The listing builds one solid part. Answer for the finished solid, in the listing's coordinates (mm). Face numbers are marked on the shaded views. Coordinates: 2 decimals unless noted, no trailing zeros. Order: outer loops, then holes, each group sorted by start corner. A loop starts at its lowest first (then second) coordinate and runs counter-clockwise, first axis right, second up. Notation, with made-up numbers: (30, 57.25) - (82, 57.25) arc R35 ccw to (82, 95.25) - close; hole circle Ø11 at (-10.5, -8.75). An arc over 180 degrees is marked (long way). Use a Markdown table: item, result. Add a question column.
Item 1: The part is cut by section C-C, the plane y = 7. Give the vertices of the cut face in (x, z), then the cut area to 3 significant figures.
Item 2: Find the intervals of material crossed by line 1 along X through (y, z) = (7.6, 32.7); line 2 along Z through (x, y) = (1.25, 9.75); line 3 along Y through (x, z) = (-4.75, 16), in increasing order.
Item 3: The part is cut by section B-B, the plane z = 28. Give the vertices of the cut face in (x, y), then the cut area to 3 significant figures.
Item 4: The mould has two halves that part along X. Classify the marked faces 1, 2, 3 and 4: released by +X, released by -X, zero draft, split by the parting line, or undercut.
Item 5: The part is cut by section A-A, the plane x = -14.5. Give the vertices of the cut face in (y, z), then the cut area to 3 significant figures.
Item 6: Flat-ended cylindrical pins translate along their axes: P1, Ø4, axis at x = -17.5, z = 34, coming from the -Y side; P2, Ø1, axis at x = -4, z = 20.5, coming from the -Y side; P3, Ø1.5, axis at x = -9.5, z = 22, coming from the -Y side. Find the tip coordinate at first contact, or state that the pin passes through.
Item 7: The part is cut by section D-D, the plane z = 12.7. Give the vertices of the cut face in (x, y), then the cut area to 3 significant figures.
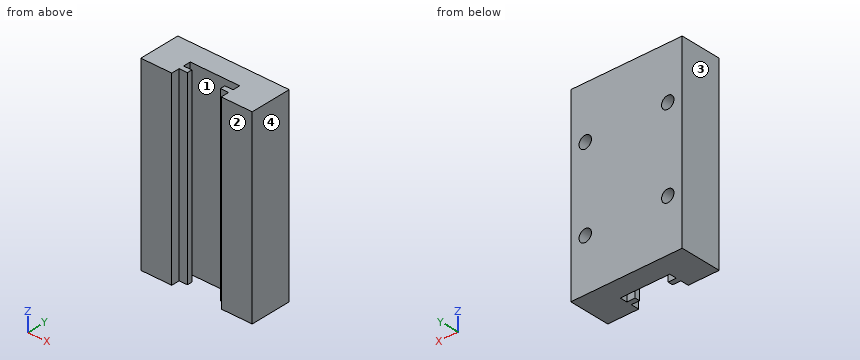
from build123d import *

# Parameters (mm, degrees)
BOSS_EXTRU_1_DEPTH      = 45.4
ESQUISSE2_R             = 1.5
ENL_V_MAT_EXTRU_1_DEPTH = 3.5


with BuildPart() as part:
    # Esquisse1 → Boss.-Extru.1 (new body)
    with BuildSketch(Plane.XY):
        Polygon((-22.795509579, 10), (4.204490421, 10), (4.204490421, 0), (-3.295509579, 0), (-3.295509579, 2), (-5.295509579, 2), (-5.295509579, 3.2), (-3.295509579, 3.2), (-3.295509579, 5), (-15.295509579, 5), (-15.295509579, 3.2), (-13.295509579, 3.2), (-13.295509579, 2), (-15.295509579, 2), (-15.295509579, 0), (-22.795509579, 0), align=None)
    extrude(amount=BOSS_EXTRU_1_DEPTH)

    # Esquisse2 → Enlèv. mat.-Extru.1 (cut)
    with BuildSketch(Plane(origin=(0, 10, 0), x_dir=(1, 0, 0), z_dir=(0, 1, 0))):
        with Locations(Location((-19.295509579, -32.7, 0), (0, 0, 270))):
            Circle(ESQUISSE2_R)
        with Locations(Location((-19.295509579, -12.7, 0), (0, 0, 270))):
            Circle(ESQUISSE2_R)
        with Locations(Location((0.704490421, -12.7, 0), (0, 0, 270))):
            Circle(ESQUISSE2_R)
        with Locations(Location((0.704490421, -32.7, 0), (0, 0, 270))):
            Circle(ESQUISSE2_R)
    extrude(amount=-ENL_V_MAT_EXTRU_1_DEPTH, mode=Mode.SUBTRACT)


solid = part.part
Solution:
| question | item | result |
|---|---|---|
| 1 | outline | (-22.8, 0) - (4.2, 0) - (4.2, 45.4) - (-22.8, 45.4) - close; hole circle Ø3 at (-19.3, 12.7); hole circle Ø3 at (-19.3, 32.7); hole circle Ø3 at (0.7, 12.7); hole circle Ø3 at (0.7, 32.7) |
| 1 | area | 1,200 mm2 |
| 2 | line 1 | x = -22.8 to -20.8, -17.8 to -0.8, 2.2 to 4.2 |
| 2 | line 2 | z = 0 to 11.3, 14.1 to 31.3, 34.1 to 45.4 |
| 2 | line 3 | y = 2 to 3.2, 5 to 10 |
| 3 | outline | (-22.8, 0) - (-15.3, 0) - (-15.3, 2) - (-13.3, 2) - (-13.3, 3.2) - (-15.3, 3.2) - (-15.3, 5) - (-3.3, 5) - (-3.3, 3.2) - (-5.3, 3.2) - (-5.3, 2) - (-3.3, 2) - (-3.3, 0) - (4.2, 0) - (4.2, 10) - (-22.8, 10) - close |
| 3 | area | 215 mm2 |
| 4 | face 1 | undercut |
| 4 | face 2 | zero draft |
| 4 | face 3 | released by -X |
| 4 | face 4 | released by +X |
| 5 | outline | (2, 0) - (3.2, 0) - (3.2, 45.4) - (2, 45.4) - close; (5, 0) - (10, 0) - (10, 45.4) - (5, 45.4) - close |
| 5 | area | 281 mm2 |
| 6 | P1 | stops at y = 0 |
| 6 | P2 | stops at y = 2 |
| 6 | P3 | stops at y = 5 |
| 7 | outline | (-22.8, 0) - (-15.3, 0) - (-15.3, 2) - (-13.3, 2) - (-13.3, 3.2) - (-15.3, 3.2) - (-15.3, 5) - (-3.3, 5) - (-3.3, 3.2) - (-5.3, 3.2) - (-5.3, 2) - (-3.3, 2) - (-3.3, 0) - (4.2, 0) - (4.2, 10) - (2.2, 10) - (2.2, 6.5) - (-0.8, 6.5) - (-0.8, 10) - (-17.8, 10) - (-17.8, 6.5) - (-20.8, 6.5) - (-20.8, 10) - (-22.8, 10) - close |
| 7 | area | 194 mm2 |
